CAD build for the part. Positions are in the model's coordinates, mm. Coordinates: 2 decimals unless noted, no trailing zeros. Loops run counter-clockwise (first coordinate to the right, second up) from the corner with the lowest first, then second, coordinate; pieces in that order, holes last. Notation, with made-up numbers: (-35, -6) -> (15, -6) arc R15 cw to (15, 14) -> close; hole circle Ø7 at (18, 36.25). An arc over 180 degrees is marked (long way). Answer as CSV lines item,"result". Start each with the question number.
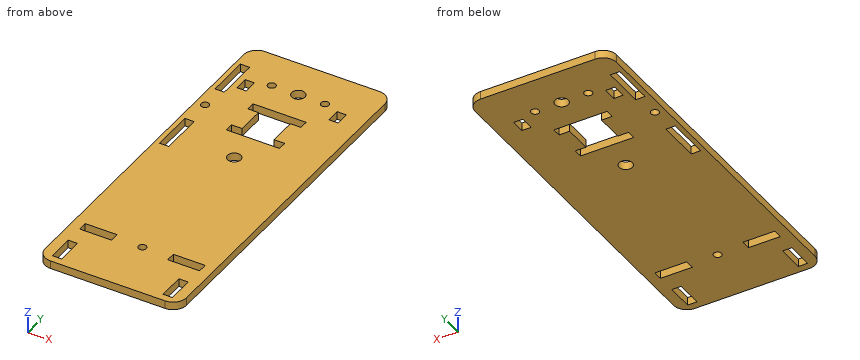
```python
from build123d import *

# Parameters (mm, degrees)
CROQUIS1_R              = 1.5
CROQUIS1_R_2            = 2.5
CROQUIS1_W              = 12
CROQUIS1_H              = 3.5
CROQUIS1_W_2            = 3.5
CROQUIS1_H_2            = 10
CROQUIS1_H_3            = 16
CROQUIS1_H_4            = 5.2
SALIENTE_EXTRUIR1_DEPTH = 3


with BuildPart() as part:
    # Croquis1 → Saliente-Extruir1 (new body)
    with BuildSketch(Plane.XY):
        with BuildLine():
            Line((21.575, -67.5), (-21.575, -67.5))
            ThreePointArc((-21.575, -67.5), (-25.110533906, -66.035533906), (-26.575, -62.5))
            Line((-26.575, -62.5), (-26.575, 62.5))
            ThreePointArc((-26.575, 62.5), (-25.110533906, 66.035533906), (-21.575, 67.5))
            Line((-21.575, 67.5), (21.575, 67.5))
            ThreePointArc((21.575, 67.5), (25.110533906, 66.035533906), (26.575, 62.5))
            Line((26.575, 62.5), (26.575, -62.5))
            ThreePointArc((26.575, -62.5), (25.110533906, -66.035533906), (21.575, -67.5))
        make_face()
        with Locations((0, -45.75)):
            Circle(CROQUIS1_R, mode=Mode.SUBTRACT)
        with Locations((-23.025, 32.3)):
            Circle(CROQUIS1_R, mode=Mode.SUBTRACT)
        with Locations((0, 52.5)):
            Circle(CROQUIS1_R_2, mode=Mode.SUBTRACT)
        with Locations((-10, 52.5)):
            Circle(CROQUIS1_R, mode=Mode.SUBTRACT)
        with Locations(Location((10, 52.5, 0), (0, 0, 180))):
            Circle(CROQUIS1_R, mode=Mode.SUBTRACT)
        with Locations(Location((0, 12.1, 0), (0, 0, 180))):
            Circle(CROQUIS1_R_2, mode=Mode.SUBTRACT)
        with Locations((-16.575, -45.75)):
            Rectangle(CROQUIS1_W, CROQUIS1_H, mode=Mode.SUBTRACT)
        with Locations((20.825, -59.7)):
            Rectangle(CROQUIS1_W_2, CROQUIS1_H_2, mode=Mode.SUBTRACT)
        with Locations((16.575, -45.75)):
            Rectangle(CROQUIS1_W, CROQUIS1_H, mode=Mode.SUBTRACT)
        with Locations((-20.825, -59.7)):
            Rectangle(CROQUIS1_W_2, CROQUIS1_H_2, mode=Mode.SUBTRACT)
        Polygon((10, 23.9), (-10, 23.9), (-10, 27.15), (-6, 27.15), (-6, 37.45), (-10, 37.45), (-10, 40.7), (10, 40.7), (10, 37.45), (6, 37.45), (6, 27.15), (10, 27.15), align=None, mode=Mode.SUBTRACT)
        with Locations((-23.025, 49.5)):
            Rectangle(CROQUIS1_W_2, CROQUIS1_H_3, mode=Mode.SUBTRACT)
        with Locations((-23.025, 14.5)):
            Rectangle(CROQUIS1_W_2, CROQUIS1_H_3, mode=Mode.SUBTRACT)
        with Locations((17.325, 48.3)):
            Rectangle(CROQUIS1_W_2, CROQUIS1_H_4, mode=Mode.SUBTRACT)
        with Locations((-17.325, 48.3)):
            Rectangle(CROQUIS1_W_2, CROQUIS1_H_4, mode=Mode.SUBTRACT)
    extrude(amount=SALIENTE_EXTRUIR1_DEPTH)


solid = part.part
```
Q1. Saw through at D-D (y = -45.75). List the corners of the cut face in (x, z) (3 decimals).
Q2. Saw through at A-A (x = 0). List the corners of the cut face in (y, z), and give its area (3 significant figures).
Q3. Pin check, flat tip, straight feed: pin 1 Ø1.5 at (x, z) = (-24, 1.5) entering from -Y. Stop position of the tip, or through.
Q4. Saw through at B-B (y = 32.3). List the corners of the cut face in (x, z) (3 decimals).
Q5. Probe probe 1 along X at (y, z) = (-62, 2.7) (3 decimals); probe 2 along X at (y, z) = (48.5, 2.6) (3 decimals); probe 3 along Y at (x, z) = (0, 2.3). List the from-to ranges inside material, lowest first. Write a range as from..to.
Q6. Saw through at C-C (y = 52.5). List the corners of the cut face in (x, z) (3 decimals), and give its area (3 significant figures).
Ans:
1,outline,"(-26.575, 0) -> (-22.575, 0) -> (-22.575, 3) -> (-26.575, 3) -> close; (-10.575, 0) -> (-1.5, 0) -> (-1.5, 3) -> (-10.575, 3) -> close; (1.5, 0) -> (10.575, 0) -> (10.575, 3) -> (1.5, 3) -> close; (22.575, 0) -> (26.575, 0) -> (26.575, 3) -> (22.575, 3) -> close"
2,outline,"(-67.5, 0) -> (-47.25, 0) -> (-47.25, 3) -> (-67.5, 3) -> close; (-44.25, 0) -> (9.6, 0) -> (9.6, 3) -> (-44.25, 3) -> close; (14.6, 0) -> (23.9, 0) -> (23.9, 3) -> (14.6, 3) -> close; (40.7, 0) -> (50, 0) -> (50, 3) -> (40.7, 3) -> close; (55, 0) -> (67.5, 0) -> (67.5, 3) -> (55, 3) -> close"
2,area,"316 mm²"
3,pin 1,"stops at y = -67.21"
4,outline,"(-26.575, 0) -> (-24.525, 0) -> (-24.525, 3) -> (-26.575, 3) -> close; (-21.525, 0) -> (-6, 0) -> (-6, 3) -> (-21.525, 3) -> close; (6, 0) -> (26.575, 0) -> (26.575, 3) -> (6, 3) -> close"
5,probe 1,"x = -26.575..-22.575, -19.075..19.075, 22.575..26.575"
5,probe 2,"x = -26.575..-24.775, -21.275..-19.075, -15.575..15.575, 19.075..26.575"
5,probe 3,"y = -67.5..-47.25, -44.25..9.6, 14.6..23.9, 40.7..50, 55..67.5"
6,outline,"(-26.575, 0) -> (-24.775, 0) -> (-24.775, 3) -> (-26.575, 3) -> close; (-21.275, 0) -> (-11.5, 0) -> (-11.5, 3) -> (-21.275, 3) -> close; (-8.5, 0) -> (-2.5, 0) -> (-2.5, 3) -> (-8.5, 3) -> close; (2.5, 0) -> (8.5, 0) -> (8.5, 3) -> (2.5, 3) -> close; (11.5, 0) -> (26.575, 0) -> (26.575, 3) -> (11.5, 3) -> close"
6,area,"116 mm²"
